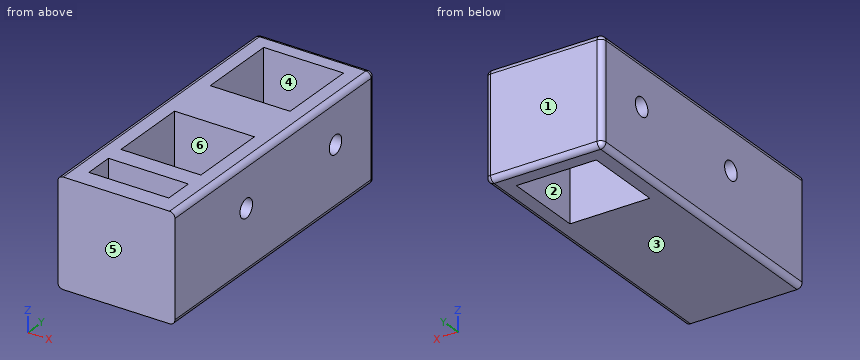
from build123d import *

# Parameters (mm, degrees)
SKETCH1_W           = 22
SKETCH1_H           = 56
SKETCH1_W_2         = 15
SKETCH1_H_2         = 15
BOSS_EXTRUDE1_DEPTH = 20
SKETCH2_W           = 15
SKETCH2_H           = 15
SKETCH2_H_2         = 5.5
CUT_EXTRUDE1_DEPTH  = 15.5
FILLET1_R           = 1
SKETCH3_R           = 1.75
CUT_EXTRUDE2_DEPTH  = 35


with BuildPart() as part:
    # Sketch1 → Boss-Extrude1 (new body)
    with BuildSketch(Plane.XY):
        with Locations((-14.096172604, 14.333947726)):
            Rectangle(SKETCH1_W, SKETCH1_H)
        with Locations((-14.096172604, 31.333947726)):
            Rectangle(SKETCH1_W_2, SKETCH1_H_2, mode=Mode.SUBTRACT)
    extrude(amount=BOSS_EXTRUDE1_DEPTH)

    # Sketch2 → Cut-Extrude1 (cut)
    with BuildSketch(Plane.XY.offset(20)):
        with Locations((-14.096172604, 6.333947726)):
            Rectangle(SKETCH2_W, SKETCH2_H)
        with Locations((-14.096172604, -7.416052274)):
            Rectangle(SKETCH2_W, SKETCH2_H_2)
    extrude(amount=-CUT_EXTRUDE1_DEPTH, mode=Mode.SUBTRACT)

    # Fillet1
    fillet1_edges = [part.edges().sort_by_distance(p)[0] for p in [
        (-3.096172604, 14.333947726, 20),
        (-14.096172604, 42.333947726, 20),
        (-25.096172604, 14.333947726, 20),
        (-14.096172604, 42.333947726, 0),
        (-3.096172604, 14.333947726, 0),
        (-25.096172604, 14.333947726, 0),
        (-25.096172604, 42.333947726, 10),
        (-3.096172604, 42.333947726, 10),
    ]]
    fillet(fillet1_edges, radius=FILLET1_R)

    # Sketch3 → Cut-Extrude2 (cut)
    with BuildSketch(Plane.ZY.offset(25.096172604)):
        with Locations(Location((11.75, 31.333947726, 0), (0, 0, 270))):
            Circle(SKETCH3_R)
        with Locations(Location((11.75, 6.333947726, 0), (0, 0, 90))):
            Circle(SKETCH3_R)
    extrude(amount=-CUT_EXTRUDE2_DEPTH, mode=Mode.SUBTRACT)


solid = part.part
For this review, take the finished solid that the model builds, in its own axes (mm). Face numbers are marked on the shaded views. A direction names the side the tool comes from. Coordinates: 2 decimals unless noted, no trailing zeros. Loops run counter-clockwise (first coordinate to the right, second up) from the corner with the lowest first, then second, coordinate; pieces in that order, holes last. Notation, with made-up numbers: (14.25, -6) -> (58.25, -6) arc R22 ccw to (58.25, 24) -> close; hole circle Ø10 at (-5.5, 33). An arc over 180 degrees is marked (long way). Write each question's results on one line, items separated by ' | '.
Q1. Machinability: for the marked faces 4, 5 and 6, which of the approach directions +Z, -Z, +X, -X, +Y, -Y give a long, thin tool a straight path to every point of the face, cutting with its end or side? Answer none if there is none.
Taken from the geometry:
face 4: +Z, -Z | face 5: +Z, -Z, +X, -X, -Y | face 6: +Z
Q2. Add section D-D, the plane x = -15.75. State the section outline as (y, z) points, then the cut area to 3 significant figures.
Taken from the geometry:
outline: (-13.67, 0) -> (23.83, 0) -> (23.83, 20) -> (13.83, 20) -> (13.83, 4.5) -> (-1.17, 4.5) -> (-1.17, 20) -> (-4.67, 20) -> (-4.67, 4.5) -> (-10.17, 4.5) -> (-10.17, 20) -> (-13.67, 20) -> close; (38.83, 0) -> (41.33, 0) arc R1 ccw to (42.33, 1) -> (42.33, 19) arc R1 ccw to (41.33, 20) -> (38.83, 20) -> close | area: 502 mm²
Q3. Mouldability with a two-part tool opening along Y and no side actions: class the marked faces 1, 2 and 3 as +Y half, -Y half, draft (parallel to the pull), parting line (faces both ways), or undercut.
Taken from the geometry:
face 1: +Y half | face 2: undercut | face 3: draft
Q4. For pin 1 Ø4 at (y, z) = (31.33, 11.75) entering from -X; pin 2 Ø4.5 at (x, y) = (-16, 9) entering from +Z, all flat-tipped, find the tip position at first contact; note any pin that passes through.
Taken from the geometry:
pin 1: x = -25.1 | pin 2: z = 4.5
Q5. Add section A-A, the plane z = 11.75. Count the separate pieces of the cut face and the enclosed holes in it, then the cut area to 3 significant figures.
Taken from the geometry:
separate pieces: 3 | enclosed holes: 1 | area: 650 mm²
Q6. Add section C-C, the plane y = 5.5. State the section outline as (x, z) points, then the cut area to 3 significant figures.
Taken from the geometry:
outline: (-25.1, 1) arc R1 ccw to (-24.1, 0) -> (-4.1, 0) arc R1 ccw to (-3.1, 1) -> (-3.1, 10.21) -> (-6.6, 10.21) -> (-6.6, 4.5) -> (-21.6, 4.5) -> (-21.6, 10.21) -> (-25.1, 10.21) -> close; (-25.1, 13.29) -> (-21.6, 13.29) -> (-21.6, 20) -> (-24.1, 20) arc R1 ccw to (-25.1, 19) -> close; (-6.6, 13.29) -> (-3.1, 13.29) -> (-3.1, 19) arc R1 ccw to (-4.1, 20) -> (-6.6, 20) -> close | area: 185 mm²
Q7. To check wall thickness, follow line 1 along Y through (x, z) = (-14.25, 7.5); line 2 along X through (y, z) = (38.5, 8.25); line 3 along Y through (x, z) = (-16, 3.75). State the ranges of each line that lie inside material, in increasing order. Write a range as [from, to].
Taken from the geometry:
line 1: [-13.67, -10.17], [-4.67, -1.17], [13.83, 23.83], [38.83, 42.33] | line 2: [-25.1, -21.6], [-6.6, -3.1] | line 3: [-13.67, 23.83], [38.83, 42.33]
Q8. Add section B-B, the plane x = -23.5. State the section outline as (y, z) points.
Taken from the geometry:
outline: (-13.67, 0) -> (41.33, 0) arc R1 ccw to (42.33, 1) -> (42.33, 19) arc R1 ccw to (41.33, 20) -> (-13.67, 20) -> close; hole circle Ø3.5 at (6.33, 11.75); hole circle Ø3.5 at (31.33, 11.75)
